Input: dimensioned drawing with shaded views. Units: mm. Origin: part minimum x, y, z. Coordinates: 2 decimals unless noted, no trailing zeros. Order: outer loops, then holes, each group sorted by start corner. A loop starts at its lowest first (then second) coordinate and runs counter-clockwise, first axis right, second up. Notation, with made-up numbers: (-25.75, -3) -> (-13.75, -3) arc R20 cw to (-13.75, 28) -> close; hole circle Ø5 at (10, -40). An arc over 180 degrees is marked (long way). Write item = value, one per line. Start each with the question number.
Item 1: Mould query, pull axis X, two halves, no side actions, for the marked faces 1 and 2. Classes: released by +X, released by -X, zero draft, split by the parting line, or undercut.
Item 2: Section query C-C (x = 180). Output: boundary loops of the cut face in (y, z), then the cut area to 3 significant figures.
Item 3: Section query D-D (z = 39.5). Output: boundary loops of the cut face in (x, y).
Item 4: Contact query for flat-ended pins moving along their axis: pin 1 (2 mm diameter, centred on x = 34.5, y = 1, fed in from -Z); pin 2 (2.5 mm diameter, centred on x = 151, y = 3.5, fed in from +Z); pin 3 (6 mm diameter, centred on x = 199, z = 16, fed in from -Y); pin 4 (0.6 mm diameter, centred on y = 5.5, z = 77, fed in from -X). Output: stop coordinate, or through.
Item 5: Section query A-A (z = 75). Output: boundary loops of the cut face in (x, y), then the cut area to 3 significant figures.
Item 6: Ray query, line 1 along Z through (x, y) = (20.5, 4); line 2 along X through (y, z) = (5.75, 75); line 3 along X through (y, z) = (0.5, 27.5). Return the intervals inside material, ascending. Write a range as [from, to].
Item 7: Section query B-B (y = 3.5). Output: boundary loops of the cut face in (x, z).
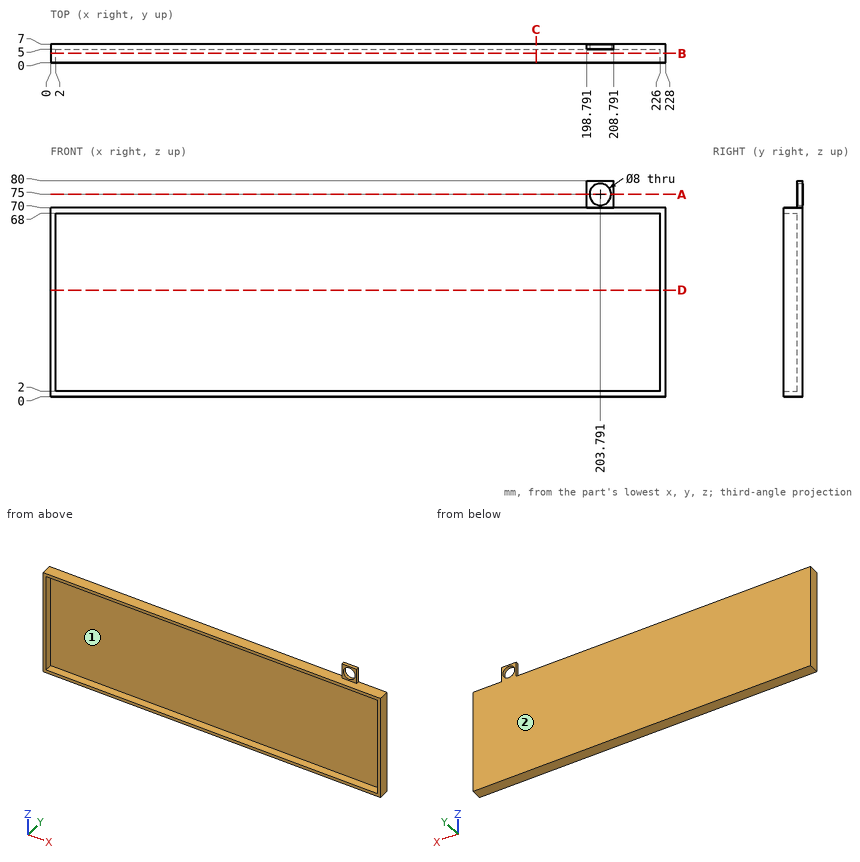
Computed:
q1.face_1 = undercut
q1.face_2 = zero draft
q2.outline = (0, 0) -> (7, 0) -> (7, 70) -> (0, 70) -> (0, 68) -> (5, 68) -> (5, 2) -> (0, 2) -> close
q2.area = 160 mm^2
q3.outline = (0, 0) -> (2, 0) -> (2, 5) -> (226, 5) -> (226, 0) -> (228, 0) -> (228, 7) -> (0, 7) -> close
q4.pin_1 = 0
q4.pin_2 = 70
q4.pin_3 = 5
q4.pin_4 = 198.79
q5.outline = (198.79, 5) -> (199.79, 5) -> (199.79, 7) -> (198.79, 7) -> close; (207.79, 5) -> (208.79, 5) -> (208.79, 7) -> (207.79, 7) -> close
q5.area = 4.00 mm^2
q6.line_1 = [0, 2], [68, 70]
q6.line_2 = [198.79, 199.79], [207.79, 208.79]
q6.line_3 = [0, 2], [226, 228]
q7.outline = (0, 0) -> (228, 0) -> (228, 70) -> (0, 70) -> close; hole (2, 2) -> (226, 2) -> (226, 68) -> (2, 68) -> close
